Build history of the part. All positions in model axes, mm. Face numbers are marked on the shaded views. A direction names the side the tool comes from. Round coordinates to 2 decimals unless told otherwise and drop trailing zeros. Loops run counter-clockwise (first coordinate to the right, second up) from the corner with the lowest first, then second, coordinate; pieces in that order, holes last. Notation, with made-up numbers: M 47.5,-16 L 55.5,-16 A15 ccw 55.5,3 Z; hole C 35,17.5 d7. An arc over 180 degrees is marked long. One line per item, written item: value.
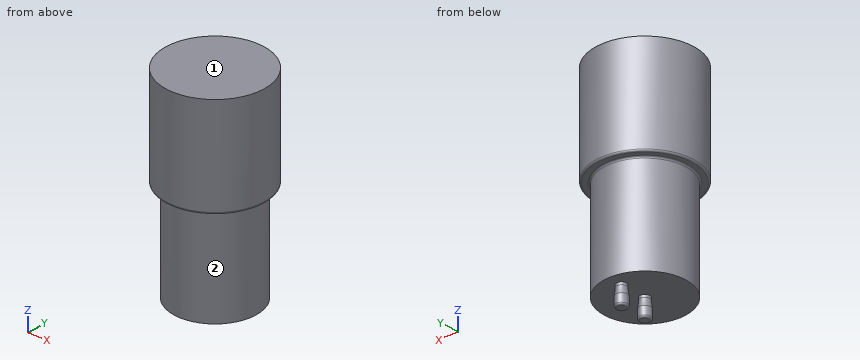
```python
from build123d import *

# Parameters (mm, degrees)
SKETCH_1_R      = 12.5
EXTRUDE_1_DEPTH = 60
SKETCH_3_R      = 1.5
EXTRUDE_2_DEPTH = 3
SKETCH_4_R      = 1.75
EXTRUDE_3_DEPTH = 3
FILLET_1_R      = 10
FILLET_2_R      = 10
FILLET_3_R      = 0.5
SKETCH_5_R      = 15
EXTRUDE_4_DEPTH = 30
FILLET_4_R      = 0.5
FILLET_5_R      = 0.5


with BuildPart() as part:
    # 草图1 → 凸台-拉伸1 (new body)
    with BuildSketch(Plane.XY):
        Circle(SKETCH_1_R)
    extrude(amount=EXTRUDE_1_DEPTH)

    # 草图3 → 凸台-拉伸2 (add)
    with BuildSketch(Plane(origin=(0, 0, 0), x_dir=(-1, 0, 0), z_dir=(0, 0, -1))):
        with Locations(Location((0, 0, 0), (0, 0, 180))):
            Circle(SKETCH_3_R)
        with Locations(Location((0, 8, 0), (0, 0, 180))):
            Circle(SKETCH_3_R)
    extrude(amount=EXTRUDE_2_DEPTH)

    # 草图4 → 凸台-拉伸3 (add)
    with BuildSketch(Plane(origin=(0, 0, -3), x_dir=(-1, 0, 0), z_dir=(0, 0, -1))):
        Circle(SKETCH_4_R)
        with Locations((0, 8)):
            Circle(SKETCH_4_R)
    extrude(amount=EXTRUDE_3_DEPTH)

    # 圆角1
    # the kernel refuses this fillet: 10 mm, written as the material it adds along each edge
    with BuildSketch(Plane(origin=(0, 8, -3), x_dir=(1, 0, 0), z_dir=(0, 1, 0))) as fillet_1_piece_1:
        with BuildLine():
            CenterArc((11.5, -2.222048604), FILLET_1_R, 167.161431859, 12.838568141)
            Line((1.75, 0), (1.5, 0))
            Line((1.5, 0), (1.5, -2.222048604))
        make_face()
    revolve(axis=Axis((0, 8, -3), (0, 0, -1)))

    # 圆角2
    # the kernel refuses this fillet: 10 mm, written as the material it adds along each edge
    with BuildSketch(Plane(origin=(0, 0, -3), x_dir=(1, 0, 0), z_dir=(0, 1, 0))) as fillet_2_piece_1:
        with BuildLine():
            CenterArc((11.5, -2.222048604), FILLET_2_R, 167.161431859, 12.838568141)
            Line((1.75, 0), (1.5, 0))
            Line((1.5, 0), (1.5, -2.222048604))
        make_face()
    revolve(axis=Axis((0, 0, -3), (0, 0, -1)))

    # 圆角3
    fillet_3_edges = [part.edges().sort_by_distance(p)[0] for p in [
        (1.75, 0, -6),
        (1.75, 8, -6),
    ]]
    fillet(fillet_3_edges, radius=FILLET_3_R)

    # 草图5 → 凸台-拉伸4 (add)
    with BuildSketch(Plane.XY.offset(60)):
        Circle(SKETCH_5_R)
    extrude(amount=-EXTRUDE_4_DEPTH)

    # 圆角4
    fillet_4_edges = [part.edges().sort_by_distance(p)[0] for p in [
        (-12.5, 0, 30),
    ]]
    fillet(fillet_4_edges, radius=FILLET_4_R)

    # 圆角5
    fillet_5_edges = [part.edges().sort_by_distance(p)[0] for p in [
        (-15, 0, 30),
    ]]
    fillet(fillet_5_edges, radius=FILLET_5_R)


solid = part.part
```
Item 1: Slice it at D-D, the plane z = 12. Give the cut face in (x, y).
Check values:
outline: C 0,0 d25
Item 2: Slice it at A-A, the plane y = 0. Give the cut face in (x, z), and give its area (3 significant figures).
Check values:
outline: M -15,30.5 A0.5 ccw -14.5,30 L -13,30 A0.5 cw -12.5,29.5 L -12.5,0 L -1.5,0 L -1.5,-0.78 A10 cw -1.75,-3 L -1.75,-5.5 A0.5 ccw -1.25,-6 L 1.25,-6 A0.5 ccw 1.75,-5.5 L 1.75,-3 A10 cw 1.5,-0.78 L 1.5,0 L 12.5,0 L 12.5,29.5 A0.5 cw 13,30 L 14.5,30 A0.5 ccw 15,30.5 L 15,60 L -15,60 Z
area: 1,670 mm2
Item 3: Slice it at C-C, the plane z = 54. Give the cut face in (x, y), and give its area (3 significant figures).
Check values:
outline: C 0,0 d30
area: 707 mm2
Item 4: Drop flat-ended pins along their axis: P1, Ø8, axis at x = 5.5, z = 20, coming from the -Y side; P2, Ø1.5, axis at y = 6, z = 31, coming from the +X side; P3, Ø2, axis at x = 2, z = 42.5, coming from the +Y side. Give the stop position or say it passes through.
Check values:
P1: stops at y = -12.41
P2: stops at x = 14.05
P3: stops at y = 14.97
Item 5: Wall check: line 1 along X through (y, z) = (0, 20); line 2 along Z through (x, y) = (-7, 0.75); line 3 along Z through (x, y) = (-1.5, -13.75). Give the ranges that are in metal, low to high.
Check values:
line 1: x = -12.5 to 12.5
line 2: z = 0 to 60
line 3: z = 30 to 60
Item 6: Which spindle directions (+Z, -Z, +X, -X, +Y, -Y) get a long thin tool onto all of the face, cutting with end or side? Do the marked faces 1 and 2. Say none if no direction does.
Check values:
face 1: +Z, +X, -X, +Y, -Y
face 2: -Z
